Geometry: final body of the model. Coordinates: model frame, mm. Give positions to 0.01 mm unless a question says otherwise; leave off trailing zeros. Write each loop counter-clockwise with the first axis right and the second up, starting at its lowest first coordinate (ties: lowest second). Pieces come first, ordered by that corner, then holes. Notation, with made-up numbers: (75, 68) -> (125, 68) arc R9 ccw to (125, 77) -> close; hole circle Ø6 at (44.25, 46.25). An arc over 180 degrees is marked (long way). Answer as a JSON object with one key per item and string values. Group by question number.
(1) Section query A-A on x = 541. Output: boundary loops of the cut face in (y, z), plus the area to 4 significant figures.
(2) Material intervals for probe 1 along Y at (x, z) = (-123, 2.5); probe 2 along Y at (x, z) = (520, 9); probe 3 along Y at (x, z) = (600, 12.45), sorted ascending.
(3) Contact query for flat-ended pins moving along their axis: pin 1 Ø3.5 at (x, y) = (598, -19) entering from -Z; pin 2 Ø11 at (x, y) = (620, 30) entering from -Z; pin 3 Ø5 at (x, y) = (128, 0.5) entering from -Z. Output: stop coordinate, or through.
from build123d import *

# Parameters (mm, degrees)
SKETCH_1_W                 = 1400
SKETCH_1_H                 = 80
EXTRUDE_1_DEPTH            = 14
SKETCH_2_W                 = 1500
SKETCH_2_H                 = 28
CUT_EXTRUDE_1_DEPTH        = 4
HOLE_WIZARD_1_D            = 6.6
HOLE_WIZARD_1_CBORE_D      = 11
HOLE_WIZARD_1_CBORE_DEPTH  = 8
PATTERN_LINEAR_1_COUNT     = 4
PATTERN_LINEAR_1_PITCH     = 200
PATTERN_LINEAR_1_COL_COUNT = 4
PATTERN_LINEAR_1_COL_PITCH = 200
HOLE_WIZARD_M8_1_D         = 6.8
PATTERN_LINEAR_2_COUNT     = 18
PATTERN_LINEAR_2_PITCH     = 80
CHAMFER_1_SIZE             = 10
CHAMFER_2_SIZE             = 1
SKETCH_9_W                 = 20
SKETCH_9_H                 = 6
CUT_EXTRUDE_2_DEPTH        = 705.695678999
HOLE_WIZARD_M8_2_D         = 6.8
CHAMFER_3_SIZE             = 1


# Some blends are built 0.0001 mm under size
with BuildPart() as part:
    # 草图1 → 凸台-拉伸1 (new body)
    with BuildSketch(Plane.XY):
        Rectangle(SKETCH_1_W, SKETCH_1_H)
    extrude(amount=EXTRUDE_1_DEPTH)

    # 草图2 → 切除-拉伸1 (cut)
    with BuildSketch(Plane(origin=(0, 0, 0), x_dir=(-1, 0, 0), z_dir=(0, 0, -1))):
        Rectangle(SKETCH_2_W, SKETCH_2_H)
    extrude(amount=-CUT_EXTRUDE_1_DEPTH, mode=Mode.SUBTRACT)

    # 打孔尺寸(%根据)内六角圆柱头螺钉的类型1 (through all)
    with Locations(Plane(origin=(0, 0, 0), x_dir=(-1, 0, 0), z_dir=(0, 0, -1))):
        with Locations((0, -20), (0, 20)):
            hole_wizard_1 = CounterBoreHole(HOLE_WIZARD_1_D / 2, HOLE_WIZARD_1_CBORE_D / 2, HOLE_WIZARD_1_CBORE_DEPTH)

    # 阵列(线性)1: 打孔尺寸(%根据)内六角圆柱头螺钉的类型1 ×4
    with Locations(*[(i * PATTERN_LINEAR_1_PITCH, 0, 0) for i in range(1, PATTERN_LINEAR_1_COUNT)]):
        add(hole_wizard_1, mode=Mode.SUBTRACT)

    # 阵列(线性)1 col: 打孔尺寸(%根据)内六角圆柱头螺钉的类型1 ×4
    with Locations(*[(-i * PATTERN_LINEAR_1_COL_PITCH, 0, 0) for i in range(1, PATTERN_LINEAR_1_COL_COUNT)]):
        add(hole_wizard_1, mode=Mode.SUBTRACT)

    # M8 螺纹孔1 (through all)
    with Locations(Plane(origin=(0, 0, 4), x_dir=(-1, 0, 0), z_dir=(0, 0, -1))):
        with Locations((-680, 0)):
            hole_wizard_m8_1 = Hole(HOLE_WIZARD_M8_1_D / 2)

    # 阵列(线性)2: M8 螺纹孔1 ×18
    with Locations(*[(-i * PATTERN_LINEAR_2_PITCH, 0, 0) for i in range(1, PATTERN_LINEAR_2_COUNT)]):
        add(hole_wizard_m8_1, mode=Mode.SUBTRACT)

    # 倒角1
    chamfer_1_edges = [part.edges().sort_by_distance(p)[0] for p in [
        (700, -40, 7),
        (-700, -40, 7),
        (-700, 40, 7),
        (700, 40, 7),
    ]]
    chamfer(chamfer_1_edges, length=CHAMFER_1_SIZE)

    # 倒角2
    # the kernel refuses this chamfer: 1 mm, written as the material it takes off along each edge
    with BuildSketch(Plane(origin=(700, 32.571682988, 0), x_dir=(-0.9996219169112968, 0, -0.027495876610586483), z_dir=(0, -1, 0)), Plane(origin=(-700, 11.428317012, 0), x_dir=(0.9996219169112968, 0, -0.027495876610586483), z_dir=(0, 1, 0))) as chamfer_2_piece_1:
        Polygon((CHAMFER_2_SIZE * 0.999621916911, -CHAMFER_2_SIZE * 0.0274958766106), (-CHAMFER_2_SIZE * 0.0274958766106, -CHAMFER_2_SIZE * 0.999621916911), (0, 0), align=None)
    extrude(amount=21.143365976, mode=Mode.SUBTRACT)
    with BuildSketch(Plane(origin=(-700, -32.571682988, 0), x_dir=(-0.027495876610582174, 0, 0.9996219169112968), z_dir=(0, 1, 0)), Plane(origin=(700, -11.428317012, 0), x_dir=(0.027495876610582174, 0, 0.9996219169112968), z_dir=(0, -1, 0))) as chamfer_2_piece_2:
        Polygon((CHAMFER_2_SIZE * 0.999621916911, CHAMFER_2_SIZE * 0.0274958766106), (-CHAMFER_2_SIZE * 0.0274958766106, CHAMFER_2_SIZE * 0.999621916911), (0, 0), align=None)
    extrude(amount=21.143365976, mode=Mode.SUBTRACT)
    with BuildSketch(Plane(origin=(-702.571682988, -14, 0), x_dir=(0, -0.9996219169112968, -0.02749587661058639), z_dir=(1, 0, 0)), Plane(origin=(702.571682988, 14, 0), x_dir=(0, 0.9996219169112968, -0.02749587661058639), z_dir=(-1, 0, 0))) as chamfer_2_piece_3:
        Polygon((CHAMFER_2_SIZE * 0.999621916911, -CHAMFER_2_SIZE * 0.0274958766106), (-CHAMFER_2_SIZE * 0.0274958766106, -CHAMFER_2_SIZE * 0.999621916911), (0, 0), align=None)
    extrude(amount=1405.143365976, mode=Mode.SUBTRACT)
    with BuildSketch(Plane(origin=(692.571682988, -40, 0), x_dir=(0, -0.02749587661058908, 0.9996219169112968), z_dir=(-1, 0, 0)), Plane(origin=(692.571682988, -40, 14), x_dir=(0, 0.9996219169112968, 0.02749587661058555), z_dir=(-1, 0, 0)), Plane(origin=(-692.571682988, 40, 0), x_dir=(0, 0.02749587661058908, 0.9996219169112968), z_dir=(1, 0, 0))) as chamfer_2_piece_4:
        Polygon((CHAMFER_2_SIZE * 0.999621916911, CHAMFER_2_SIZE * 0.0274958766106), (-CHAMFER_2_SIZE * 0.0274958766106, CHAMFER_2_SIZE * 0.999621916911), (0, 0), align=None)
    extrude(amount=1385.143365976, mode=Mode.SUBTRACT)
    with BuildSketch(Plane(origin=(701.81845448, -28.18154552, 0), x_dir=(0.01944252080600517, -0.01944252080600517, 0.9996219169112972), z_dir=(-0.7071067811865476, -0.7071067811865476, 0)), Plane(origin=(701.81845448, -28.18154552, 14), x_dir=(-0.7068394360706735, 0.7068394360706735, 0.027495876610585897), z_dir=(-0.7071067811865476, -0.7071067811865476, 0)), Plane(origin=(-688.18154552, 41.81845448, 14), x_dir=(-0.019442520805986165, 0.019442520805986165, -0.9996219169112978), z_dir=(-0.7071067811865476, -0.7071067811865476, 0)), Plane(origin=(-688.18154552, 41.81845448, 0), x_dir=(0.7068394360706736, -0.7068394360706736, -0.02749587661058688), z_dir=(-0.7071067811865476, -0.7071067811865476, 0))) as chamfer_2_piece_5:
        Polygon((CHAMFER_2_SIZE * 0.999621916911, CHAMFER_2_SIZE * 0.0274958766106), (-CHAMFER_2_SIZE * 0.0274958766106, CHAMFER_2_SIZE * 0.999621916911), (0, 0), align=None)
    extrude(amount=19.2855016, mode=Mode.SUBTRACT)
    with BuildSketch(Plane(origin=(-701.81845448, -28.18154552, 0), x_dir=(-0.01944252080600517, -0.01944252080600517, 0.9996219169112972), z_dir=(0.7071067811865476, -0.7071067811865476, 0)), Plane(origin=(688.18154552, 41.81845448, 14), x_dir=(0.019442520805986165, 0.019442520805986165, -0.9996219169112978), z_dir=(0.7071067811865476, -0.7071067811865476, 0)), Plane(origin=(-701.81845448, -28.18154552, 14), x_dir=(0.7068394360706735, 0.7068394360706735, 0.027495876610585897), z_dir=(0.7071067811865476, -0.7071067811865476, 0)), Plane(origin=(688.18154552, 41.81845448, 0), x_dir=(-0.7068394360706736, -0.7068394360706736, -0.02749587661058688), z_dir=(0.7071067811865476, -0.7071067811865476, 0))) as chamfer_2_piece_6:
        Polygon((CHAMFER_2_SIZE * 0.999621916911, -CHAMFER_2_SIZE * 0.0274958766106), (-CHAMFER_2_SIZE * 0.0274958766106, -CHAMFER_2_SIZE * 0.999621916911), (0, 0), align=None)
    extrude(amount=19.2855016, mode=Mode.SUBTRACT)
    with BuildSketch(Plane(origin=(-700, -32.571682988, 14), x_dir=(0.9996219169112968, 0, 0.02749587661058574), z_dir=(0, 1, 0)), Plane(origin=(700, 32.571682988, 14), x_dir=(-0.9996219169112968, 0, 0.02749587661058574), z_dir=(0, -1, 0))) as chamfer_2_piece_7:
        Polygon((CHAMFER_2_SIZE * 0.999621916911, CHAMFER_2_SIZE * 0.0274958766106), (-CHAMFER_2_SIZE * 0.0274958766106, CHAMFER_2_SIZE * 0.999621916911), (0, 0), align=None)
    extrude(amount=65.143365976, mode=Mode.SUBTRACT)
    with BuildSketch(Plane(origin=(-692.571682988, 40, 14), x_dir=(0, 0.0274958766105891, -0.9996219169112968), z_dir=(1, 0, 0))) as chamfer_2_piece_8:
        Polygon((CHAMFER_2_SIZE * 0.999621916911, -CHAMFER_2_SIZE * 0.0274958766106), (-CHAMFER_2_SIZE * 0.0274958766106, -CHAMFER_2_SIZE * 0.999621916911), (0, 0), align=None)
    extrude(amount=1385.143365976, mode=Mode.SUBTRACT)

    # 草图9 → 切除-拉伸2 (cut, through all)
    with BuildSketch(Plane.XZ.offset(40)):
        with Locations((-620, 0)):
            Rectangle(SKETCH_9_W, SKETCH_9_H)
    cut_extrude_2 = extrude(amount=-CUT_EXTRUDE_2_DEPTH, mode=Mode.SUBTRACT)

    # M8 螺纹孔2 (through all)
    with Locations(Plane(origin=(0, 0, 3), x_dir=(-1, 0, 0), z_dir=(0, 0, -1))):
        with Locations((620, -30), (620, 30)):
            hole_wizard_m8_2 = Hole(HOLE_WIZARD_M8_2_D / 2)

    # 镜向1: 切除-拉伸2, M8 螺纹孔2 across plane
    add(cut_extrude_2.mirror(Plane(origin=(0, 0, 0), x_dir=(0, 0, 1), z_dir=(1, 0, 0))), mode=Mode.SUBTRACT)
    add(hole_wizard_m8_2.mirror(Plane(origin=(0, 0, 0), x_dir=(0, 0, 1), z_dir=(1, 0, 0))), mode=Mode.SUBTRACT)

    # 倒角3
    chamfer_3_edges = [part.edges().sort_by_distance(p)[0] for p in [
        (-610, 39.5, 0.5),
        (-630, 39.5, 0.5),
        (-620, -14, 3),
        (-620, 14, 3),
        (-620, 40, 3),
        (-630, -14, 2),
        (-630, -27, 0),
        (-630, 14, 2),
        (-630, 40, 2),
        (-630, 27, 0),
        (-610, -14, 2),
        (-610, -27, 0),
        (-610, 14, 2),
        (-610, 27, 0),
        (-610, 40, 2),
        (-630, 14.5, 0.5),
        (-630, -39.5, 0.5),
        (-630, -14.5, 0.5),
        (-610, -14.5, 0.5),
        (-610, -39.5, 0.5),
        (-610, 14.5, 0.5),
        (-610, -40, 2),
        (-620, -40, 3),
        (-630, -40, 2),
        (610, 39.5, 0.5),
        (630, 39.5, 0.5),
        (620, -14, 3),
        (620, -40, 3),
        (630, -40, 2),
        (630, -39.5, 0.5),
        (630, -14.5, 0.5),
        (630, 14.5, 0.5),
        (610, -14.5, 0.5),
        (610, -39.5, 0.5),
        (610, -40, 2),
        (610, 14.5, 0.5),
        (630, -14, 2),
        (630, -27, 0),
        (630, 27, 0),
        (630, 14, 2),
        (610, -14, 2),
        (610, 14, 2),
        (610, 27, 0),
        (610, -27, 0),
        (620, 14, 3),
        (630, 40, 2),
        (610, 40, 2),
        (620, 40, 3),
    ]]
    chamfer(chamfer_3_edges, length=CHAMFER_3_SIZE - 0.0001)  # a hair under: the kernel refuses the full size


solid = part.part
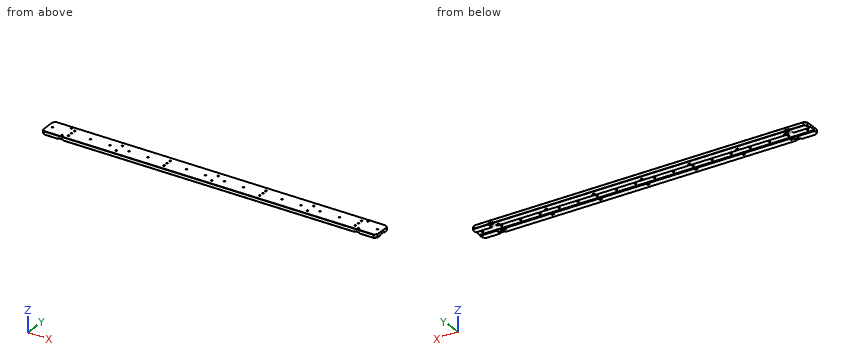
Answer list:
{
 "1": {"outline": "(-40, 1) -> (-39, 0) -> (-15, 0) -> (-14, 1) -> (-14, 4) -> (14, 4) -> (14, 1) -> (15, 0) -> (39, 0) -> (40, 1) -> (40, 13) -> (39, 14) -> (-39, 14) -> (-40, 13) -> close", "area": "1,005 mm2"},
 "2": {"probe 1": "-40 to -14, 14 to 40", "probe 2": "-40 to -3.4, 3.4 to 40", "probe 3": "-40 to -23.3, -16.7 to -3.4, 3.4 to 16.7, 23.3 to 40"},
 "3": {"pin 1": "z = 8", "pin 2": "z = 3", "pin 3": "z = 4"}
}
